For this review, take the finished solid that the model builds, in its own axes (mm). Face numbers are marked on the shaded views. A direction names the side the tool comes from. Round coordinates to 2 decimals unless told otherwise and drop trailing zeros. Put each result on its own line as item: value.
from build123d import *

# Parameters (mm, degrees)
SKETCH_1_W                         = 40
SKETCH_1_H                         = 40
EXTRUDE_1_DEPTH                    = 6
SKETCH_2_R                         = 3
CUT_EXTRUDE_1_DEPTH                = 6
PATTERN_LINEAR_1_COUNT             = 2
PATTERN_LINEAR_1_PITCH             = 20
CHAMFER_1_SIZE                     = 6
SKETCH_3_W                         = 34
SKETCH_3_H                         = 3
EXTRUDE_2_DEPTH                    = 34
CHAMFER_2_SIZE                     = 34
PATTERN_LINEAR_2_COUNT             = 2
PATTERN_LINEAR_2_PITCH             = 37
CHAMFER_2_OF_PATTERN_LINEAR_2_SIZE = 34
SHELL_START                        = 2.8
SHELL_3_OUTLINE_W                  = 3.2
SHELL_3_OUTLINE_H                  = 34.4
SHELL_3_DEPTH                      = 34.4
SHELL_3_2_OUTLINE_W                = 31.2
SHELL_3_2_OUTLINE_H                = 34.4
SHELL_3_2_OUTLINE_R                = 5.8
SHELL_3_2_DEPTH                    = 3.2
SHELL_START_2                      = -8.776349614
SHELL_3_3_OUTLINE_R                = 5.8
SHELL_3_3_OUTLINE_R_2              = 3
SHELL_3_3_DEPTH                    = 3.2
SHELL_START_3                      = -16
SHELL_3_4_DEPTH                    = 37
CHAMFER_5_SIZE                     = 5.67128182
CHAMFER_5_SIZE_2                   = 1
CHAMFER_6_SIZE                     = 5.67128182
CHAMFER_6_SIZE_2                   = 1
CHAMFER_7_SIZE                     = 2.7
CHAMFER_7_SIZE_2                   = 4.67653718


with BuildPart() as part:
    # Эскиз1 → Бобышка-Вытянуть1 (new body)
    with BuildSketch(Plane.XY):
        with Locations((-22.776349614, 2.36503856)):
            Rectangle(SKETCH_1_W, SKETCH_1_H)
    extrude(amount=EXTRUDE_1_DEPTH)

    # Эскиз2 → Вырез-Вытянуть1 (cut)
    with BuildSketch(Plane.XY.offset(6)):
        with Locations((-32.776349614, 12.36503856)):
            Circle(SKETCH_2_R)
    cut_extrude_1 = extrude(amount=-CUT_EXTRUDE_1_DEPTH, mode=Mode.SUBTRACT)

    # Линейный массив1: Вырез-Вытянуть1 ×2
    with Locations(*[(0, -i * PATTERN_LINEAR_1_PITCH, 0) for i in range(1, PATTERN_LINEAR_1_COUNT)]):
        add(cut_extrude_1, mode=Mode.SUBTRACT)

    # Фаска1
    chamfer_1_edges = [part.edges().sort_by_distance(p)[0] for p in [
        (-2.776349614, 2.36503856, 6),
    ]]
    chamfer(chamfer_1_edges, length=CHAMFER_1_SIZE - 0.0001)  # a hair under: the kernel refuses the full size

    # Зеркальное отражение1: part across plane


with BuildPart() as part_1:
    add(part.part)
    add(part.part.mirror(Plane(origin=(-8.776349614, 0, 6), x_dir=(-0.7071067811865465, 0, 0.7071067811865486), z_dir=(0.7071067811865488, 0, 0.7071067811865464))))

    # Эскиз3 → Бобышка-Вытянуть2 (add)
    with BuildSketch(Plane.XY.offset(6)):
        with Locations((-25.776349614, 20.86503856)):
            Rectangle(SKETCH_3_W, SKETCH_3_H)
    extrude_2 = extrude(amount=EXTRUDE_2_DEPTH)

    # Фаска2
    chamfer_2_edges = [part_1.edges().sort_by_distance(p)[0] for p in [
        (-42.776349614, 20.86503856, 40),
    ]]
    chamfer(chamfer_2_edges, length=CHAMFER_2_SIZE)

    # Линейный массив2: Бобышка-Вытянуть2 ×2
    with Locations(*[(0, -i * PATTERN_LINEAR_2_PITCH, 0) for i in range(1, PATTERN_LINEAR_2_COUNT)]):
        add(extrude_2)

    # Фаска2 of Линейный массив2
    chamfer_2_of_pattern_linear_2_edges = [part_1.edges().sort_by_distance(p)[0] for p in [
        (-42.776349614, -16.13496144, 40),
    ]]
    chamfer(chamfer_2_of_pattern_linear_2_edges, length=CHAMFER_2_OF_PATTERN_LINEAR_2_SIZE)

    # Оболочка3: read off the stored shape, not the designer's step
    # Оболочка3 outline → Оболочка3 (cut)
    with BuildSketch(Plane.XY.offset(SHELL_START)):
        with Locations((-7.176349614, 2.36503856)):
            Rectangle(SHELL_3_OUTLINE_W, SHELL_3_OUTLINE_H)
    extrude(amount=SHELL_3_DEPTH, mode=Mode.SUBTRACT)

    # Shell 3 2 outline → Shell 3 2 (cut)
    with BuildSketch(Plane.XY.offset(SHELL_START)):
        with Locations((-24.376349614, 2.36503856)):
            Rectangle(SHELL_3_2_OUTLINE_W, SHELL_3_2_OUTLINE_H)
        with Locations((-32.776349614, -7.63496144)):
            Circle(SHELL_3_2_OUTLINE_R, mode=Mode.SUBTRACT)
        with Locations((-32.776349614, 12.36503856)):
            Circle(SHELL_3_2_OUTLINE_R, mode=Mode.SUBTRACT)
    extrude(amount=SHELL_3_2_DEPTH, mode=Mode.SUBTRACT)

    # Shell 3 3 outline → Shell 3 3 (add)
    # profile 1 of 2: a face of its own
    with BuildSketch(Plane.YZ.offset(SHELL_START_2)):
        with Locations((12.36503856, 30)):
            Circle(SHELL_3_3_OUTLINE_R)
        with Locations((12.36503856, 30)):
            Circle(SHELL_3_3_OUTLINE_R_2, mode=Mode.SUBTRACT)
    # profile 2 of 2: a face of its own
    with BuildSketch(Plane.YZ.offset(SHELL_START_2)):
        with Locations((-7.63496144, 30)):
            Circle(SHELL_3_3_OUTLINE_R)
        with Locations((-7.63496144, 30)):
            Circle(SHELL_3_3_OUTLINE_R_2, mode=Mode.SUBTRACT)
    extrude(amount=SHELL_3_3_DEPTH)

    # Shell 3 4 outline → Shell 3 4 (add)
    with BuildSketch(Plane(origin=(0, 0, 0), x_dir=(1, 0, 0), z_dir=(0, 1, 0)).offset(SHELL_START_3)):
        Polygon((-39.976349614, -4.840202025), (-39.976349614, -6), (-38.81655164, -6), align=None)
        Polygon((-7.61655164, -37.2), (-8.776349614, -36.040202025), (-8.776349614, -37.2), align=None)
    extrude(amount=SHELL_3_4_DEPTH)

    # Фаска5
    # the kernel refuses this chamfer: 5.67128182, 1 mm, written as the material it takes off along each edge
    with BuildSketch(Plane(origin=(-8.776349614, 12.36503856, 30), x_dir=(0, 1, 0), z_dir=(0, 0, -1))) as chamfer_5_piece_1_section:
        Polygon((5.8, CHAMFER_5_SIZE), (5.8 - CHAMFER_5_SIZE_2, 0), (5.8, 0), align=None)
    chamfer_5_piece_1 = revolve(axis=Axis((-8.776349614, 12.36503856, 30), (1, 0, 0)), mode=Mode.PRIVATE)
    chamfer_5_piece_1 = split(chamfer_5_piece_1, bisect_by=Plane(origin=(-5.576349614, 12.36503856, 30), z_dir=(-1, 0, 0)), keep=Keep.TOP, mode=Mode.PRIVATE)
    add(chamfer_5_piece_1, mode=Mode.SUBTRACT)
    with BuildSketch(Plane(origin=(-8.776349614, -7.63496144, 30), x_dir=(0, 1, 0), z_dir=(0, 0, -1))) as chamfer_5_piece_2_section:
        Polygon((5.8 - CHAMFER_5_SIZE_2, 0), (5.8, CHAMFER_5_SIZE), (5.8, 0), align=None)
    chamfer_5_piece_2 = revolve(axis=Axis((-8.776349614, -7.63496144, 30), (1, 0, 0)), mode=Mode.PRIVATE)
    chamfer_5_piece_2 = split(chamfer_5_piece_2, bisect_by=Plane(origin=(-5.576349614, -7.63496144, 30), z_dir=(-1, 0, 0)), keep=Keep.TOP, mode=Mode.PRIVATE)
    add(chamfer_5_piece_2, mode=Mode.SUBTRACT)

    # Фаска6
    # the kernel refuses this chamfer: 5.67128182, 1 mm, written as the material it takes off along each edge
    with BuildSketch(Plane(origin=(-32.776349614, -7.63496144, 6), x_dir=(1, 0, 0), z_dir=(0, -1, 0))) as chamfer_6_piece_1_section:
        Polygon((5.8, -CHAMFER_6_SIZE), (5.8 - CHAMFER_6_SIZE_2, 0), (5.8, 0), align=None)
    chamfer_6_piece_1 = revolve(axis=Axis((-32.776349614, -7.63496144, 6), (0, 0, 1)), mode=Mode.PRIVATE)
    chamfer_6_piece_1 = split(chamfer_6_piece_1, bisect_by=Plane(origin=(-32.776349614, -7.63496144, 2.8), z_dir=(0, 0, 1)), keep=Keep.TOP, mode=Mode.PRIVATE)
    add(chamfer_6_piece_1, mode=Mode.SUBTRACT)
    with BuildSketch(Plane(origin=(-32.776349614, 12.36503856, 6), x_dir=(1, 0, 0), z_dir=(0, -1, 0))) as chamfer_6_piece_2_section:
        Polygon((5.8, -CHAMFER_6_SIZE), (5.8 - CHAMFER_6_SIZE_2, 0), (5.8, 0), align=None)
    chamfer_6_piece_2 = revolve(axis=Axis((-32.776349614, 12.36503856, 6), (0, 0, 1)), mode=Mode.PRIVATE)
    chamfer_6_piece_2 = split(chamfer_6_piece_2, bisect_by=Plane(origin=(-32.776349614, 12.36503856, 2.8), z_dir=(0, 0, 1)), keep=Keep.TOP, mode=Mode.PRIVATE)
    add(chamfer_6_piece_2, mode=Mode.SUBTRACT)

    # Фаска7
    # the kernel refuses this chamfer: 4.67653718, 2.7 mm, written as the material it adds along each edge
    with BuildSketch(Plane(origin=(-39.976349614, 19.56503856, 2.8), x_dir=(0, 0, 1), z_dir=(0, -1, 0))) as chamfer_7_piece_1_section:
        Polygon((CHAMFER_7_SIZE, 0), (0, -CHAMFER_7_SIZE_2), (0, 0), align=None)
    chamfer_7_piece_1 = extrude(amount=34.4, mode=Mode.PRIVATE)
    chamfer_7_piece_1 = chamfer_7_piece_1 - Plane(origin=(-32.776349614, -7.63496144, 2.8), x_dir=(1, 0, 0), z_dir=(0, 0, 1)) * Cylinder(3, 88, mode=Mode.PRIVATE)
    chamfer_7_piece_1 = chamfer_7_piece_1 - Plane(origin=(-32.776349614, 12.36503856, 2.8), x_dir=(1, 0, 0), z_dir=(0, 0, 1)) * Cylinder(3, 88, mode=Mode.PRIVATE)
    add(chamfer_7_piece_1)
    with BuildSketch(Plane(origin=(-5.576349614, -14.83496144, 37.2), x_dir=(-1, 0, 0), z_dir=(0, 1, 0))) as chamfer_7_piece_2_section:
        Polygon((CHAMFER_7_SIZE, 0), (0, -CHAMFER_7_SIZE_2), (0, 0), align=None)
    chamfer_7_piece_2 = extrude(amount=34.4, mode=Mode.PRIVATE)
    chamfer_7_piece_2 = chamfer_7_piece_2 - Plane(origin=(-5.576349614, -7.63496144, 30), x_dir=(0, 0, -1), z_dir=(-1, 0, 0)) * Cylinder(3, 88, mode=Mode.PRIVATE)
    chamfer_7_piece_2 = chamfer_7_piece_2 - Plane(origin=(-5.576349614, 12.36503856, 30), x_dir=(0, 0, -1), z_dir=(-1, 0, 0)) * Cylinder(3, 88, mode=Mode.PRIVATE)
    add(chamfer_7_piece_2)


solid = part_1.part
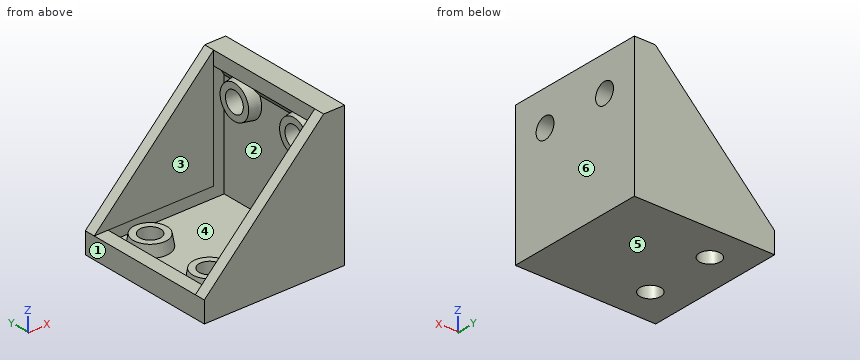
(1) To check wall thickness, follow L1, parallel to Y at x = -13, z = 7; L2, parallel to Y at x = -6.75, z = 30; L3, parallel to Z at x = -6.5, y = -5. State the ranges of each line that lie inside material, in increasing order.
A:
L1: y = -17.63 to -14.63, 19.37 to 22.37
L2: y = -17.63 to -14.83, -12.79 to -10.63, -4.63 to -2.48, 7.21 to 9.37, 15.37 to 17.52, 19.57 to 22.37
L3: z = 0 to 2.8, 25.52 to 28.57, 31.43 to 40
(2) Add section A-A on x = -30.5. State how many separate pieces and enclosed holes the cut face has, then the cut area to 3 significant figures.
A:
separate pieces: 3
enclosed holes: 0
area: 215 mm2
(3) For the marked faces 1, 2 and 3, list the 3-axis set-ups (+Z, -Z, +X, -X, +Y, -Y) from which the entire face can be reached by the end or side of a thin tool; tool diameter is ignored.
A:
face 1: +Z, -Z, -X, +Y, -Y
face 2: none
face 3: +Z, -X
(4) Insertion check: pin 1 Ø4 at (y, z) = (-5, 12.5) entering from -X; pin 2 Ø3 at (x, y) = (-14.5, -0.5) entering from +Z; pin 3 Ø9.5 at (y, z) = (-7.63, 30) entering from +X; pin 4 Ø5 at (y, z) = (12.37, 30) entering from -X (1 decimal). Each pin has a flat end and moves straight along its axis. Give the tip position at first contact, or say it passes through.
A:
pin 1: stops at x = -5.58
pin 2: stops at z = 2.8
pin 3: stops at x = -2.78
pin 4: passes through
(5) Draft analysis for pull direction X (two halves, no side actions). For the marked faces 4, 5 and 6, state which applies: released by +X, released by -X, zero draft, split by the parting line, or undercut.
A:
face 4: undercut
face 5: zero draft
face 6: released by +X
